```python
from build123d import *

# Parameters (mm, degrees)
F0_R         = 2.8
F1_DEPTH     = 11
F3_DEPTH     = 2
F5_DEPTH     = 0.5
F6_DEPTH     = 0.5
F7_R         = 0.8
F8_T4_DEPTH  = 7.176254213
F8_S5_R      = 2.8
F8_T6_DEPTH  = 5
F8_T10_DEPTH = 7.240123034
F8_S11_R     = 2.8
F8_T12_DEPTH = 5
F8_T16_DEPTH = 10.9265531961
F8_S17_R     = 2.8
F8_T18_DEPTH = 7
F8_T24_DEPTH = 10.862684375
F8_S25_R     = 2.8
F8_T26_DEPTH = 7
F9_R         = 0.8


# Not quite as in the source:
# - a fillet or chamfer that OpenCascade refuses, or shapes differently, is made with other operations: its cross-section is extruded or revolved along the edge and cut away or added


with BuildPart() as f1:
    # F0 (on Top) → F1 (new body)
    with BuildSketch(Plane.XY):
        Polygon((4.8497422612, -8.4), (9.6994845224, 0), (4.8497422612, 8.4), (-4.8497422612, 8.4), (-9.6994845224, 0), (-4.8497422612, -8.4), align=None)
        with Locations((-0.031784919, 0.0747148006)):
            Circle(F0_R, mode=Mode.SUBTRACT)
    extrude(amount=F1_DEPTH)

    # F2 (on Top) → F3 (cut)
    with BuildSketch(Plane.XY):
        with BuildLine():
            Line((-6, 1.1), (-6, -1.1))
            Line((-6, -1.1), (-3.585038354, -1.1))
            ThreePointArc((-3.585038354, -1.1), (-3.75, 0), (-3.585038354, 1.1))
            Line((-3.585038354, 1.1), (-6, 1.1))
        make_face()
        with BuildLine():
            ThreePointArc((-3.585038354, 1.1), (-3.75, 0), (-3.585038354, -1.1))
            Line((-3.585038354, -1.1), (3.585038354, -1.1))
            ThreePointArc((3.585038354, -1.1), (3.7085302903, -0.556150237), (3.75, 0))
            ThreePointArc((3.75, 0), (3.7085302903, 0.556150237), (3.585038354, 1.1))
            Line((3.585038354, 1.1), (-3.585038354, 1.1))
        make_face()
        with BuildLine():
            ThreePointArc((3.75, 0), (3.7085302903, -0.556150237), (3.585038354, -1.1))
            Line((3.585038354, -1.1), (6, -1.1))
            Line((6, -1.1), (6, 1.1))
            Line((6, 1.1), (3.585038354, 1.1))
            ThreePointArc((3.585038354, 1.1), (3.7085302903, 0.556150237), (3.75, 0))
        make_face()
    extrude(amount=F3_DEPTH, mode=Mode.SUBTRACT)

    # F4 (on face) → F5 (join)
    with BuildSketch(Plane(origin=(0, 0, 0), x_dir=(1, 0, 0), z_dir=(0, 0, -1))):
        with BuildLine():
            Line((2.509876966, 1.1), (3.585038354, 1.1))
            ThreePointArc((3.585038354, 1.1), (0, 3.75), (-3.585038354, 1.1))
            Line((-3.585038354, 1.1), (-2.5734468039, 1.1))
            ThreePointArc((-2.5734468039, 1.1), (-0.031784919, 2.7252851994), (2.509876966, 1.1))
        make_face()
    extrude(amount=F5_DEPTH)

    # F4 (on face) → F6 (join)
    with BuildSketch(Plane(origin=(0, 0, 0), x_dir=(1, 0, 0), z_dir=(0, 0, -1))):
        with BuildLine():
            ThreePointArc((-3.585038354, -1.1), (0, -3.75), (3.585038354, -1.1))
            Line((3.585038354, -1.1), (2.573745787, -1.1))
            ThreePointArc((2.573745787, -1.1), (-0.031784919, -2.8747148006), (-2.637315625, -1.1))
            Line((-2.637315625, -1.1), (-3.585038354, -1.1))
        make_face()
    extrude(amount=F6_DEPTH)

    # F7
    f7_edges = [f1.edges().sort_by_distance(p)[0] for p in [
        (-0.031785, 2.874715, -0.5),
        (-0.031785, -2.725285, -0.5),
    ]]
    fillet(f7_edges, radius=F7_R)

    # F8: fillet of radius 1.5 on 4 edges, made by hand


with BuildPart() as f8_tool2:
    # F8_s3 → F8_t4 (new body)
    with BuildSketch(Plane.YZ.offset(6)):
        with BuildLine():
            ThreePointArc((1.1, 0.5), (0.6606601718, 1.5606601718), (-0.4, 2))
            Line((-0.4, 2), (1.1, 2))
            Line((1.1, 2), (1.1, 0.5))
        make_face()
    extrude(amount=-F8_T4_DEPTH)

    # F8_s5 → F8_t6 (cut, symmetric)
    with BuildSketch(Plane.XY.offset(1.2)):
        with Locations((-0.031784919, 0.0747148006)):
            Circle(F8_S5_R)
    extrude(amount=F8_T6_DEPTH, both=True, mode=Mode.SUBTRACT)


with BuildPart() as f1_1:
    add(f1.part)

    # F8_t1: union F8_tool2
    add(f8_tool2.part)


with BuildPart() as f8_tool8:
    # F8_s9 → F8_t10 (new body)
    with BuildSketch(Plane.YZ.offset(-1.240123034)):
        with BuildLine():
            ThreePointArc((0.4, 2), (-0.6606601718, 1.5606601718), (-1.1, 0.5))
            Line((-1.1, 0.5), (-1.1, 2))
            Line((-1.1, 2), (0.4, 2))
        make_face()
    extrude(amount=F8_T10_DEPTH)

    # F8_s11 → F8_t12 (cut, symmetric)
    with BuildSketch(Plane.XY.offset(1.2)):
        with Locations((-0.031784919, 0.0747148006)):
            Circle(F8_S11_R)
    extrude(amount=F8_T12_DEPTH, both=True, mode=Mode.SUBTRACT)


with BuildPart() as f1_2:
    add(f1_1.part)

    # F8_t7: union F8_tool8
    add(f8_tool8.part)


with BuildPart() as f8_tool14:
    # F8_s15 → F8_t16 (new body)
    with BuildSketch(Plane.YZ.offset(-9.75)):
        with BuildLine():
            ThreePointArc((0.4, 2), (-0.6606601718, 1.5606601718), (-1.1, 0.5))
            Line((-1.1, 0.5), (-1.1, 2))
            Line((-1.1, 2), (0.4, 2))
        make_face()
    extrude(amount=F8_T16_DEPTH)

    # F8_s17 → F8_t18 (cut, symmetric)
    with BuildSketch(Plane.XY.offset(1.2)):
        with Locations((-0.031784919, 0.0747148006)):
            Circle(F8_S17_R)
    extrude(amount=F8_T18_DEPTH, both=True, mode=Mode.SUBTRACT)

    split(bisect_by=Plane(origin=(-7.2746133918, -4.2, 0), x_dir=(0, 0, 1), z_dir=(0.8660254038, 0.5, 0)), keep=Keep.TOP)

    split(bisect_by=Plane(origin=(-7.2746133918, 4.2, 0), x_dir=(0, 0, 1), z_dir=(0.8660254038, -0.5, 0)), keep=Keep.TOP)


with BuildPart() as f1_3:
    add(f1_2.part)

    # F8_t13: union F8_tool14
    add(f8_tool14.part)


with BuildPart() as f8_tool22:
    # F8_s23 → F8_t24 (new body)
    with BuildSketch(Plane.YZ.offset(1.112684375)):
        with BuildLine():
            ThreePointArc((1.1, 0.5), (0.6606601718, 1.5606601718), (-0.4, 2))
            Line((-0.4, 2), (1.1, 2))
            Line((1.1, 2), (1.1, 0.5))
        make_face()
    extrude(amount=-F8_T24_DEPTH)

    # F8_s25 → F8_t26 (cut, symmetric)
    with BuildSketch(Plane.XY.offset(1.2)):
        with Locations((-0.031784919, 0.0747148006)):
            Circle(F8_S25_R)
    extrude(amount=F8_T26_DEPTH, both=True, mode=Mode.SUBTRACT)

    split(bisect_by=Plane(origin=(-7.2746133918, -4.2, 0), x_dir=(0, 0, 1), z_dir=(0.8660254038, 0.5, 0)), keep=Keep.TOP)

    split(bisect_by=Plane(origin=(-7.2746133918, 4.2, 0), x_dir=(0, 0, 1), z_dir=(0.8660254038, -0.5, 0)), keep=Keep.TOP)


with BuildPart() as f1_4:
    add(f1_3.part)

    # F8_t21: union F8_tool22
    add(f8_tool22.part)

    # F9
    f9_edges = [f1_4.edges().sort_by_distance(p)[0] for p in [
        (0, -8.4, 11),
        (7.274613, -4.2, 11),
        (7.274613, 4.2, 11),
        (0, 8.4, 11),
        (-7.274613, 4.2, 11),
        (-7.274613, -4.2, 11),
    ]]
    fillet(f9_edges, radius=F9_R)


solid = f1_4.part
```
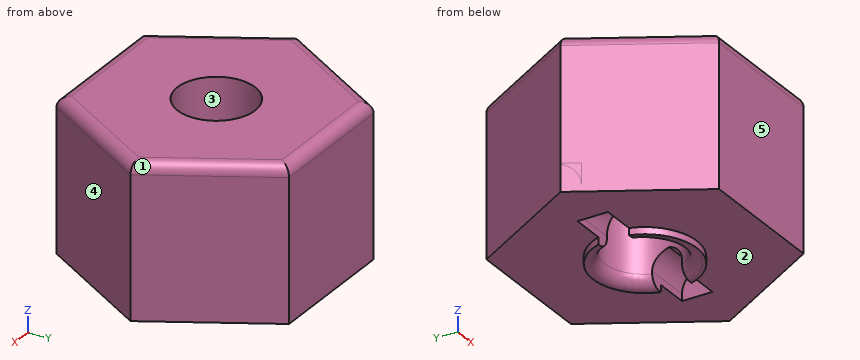
Could you check a few things on this model? Use its own coordinates, in mm. Face numbers are marked on the shaded views. A direction names the side the tool comes from. Round coordinates to 2 decimals unless told otherwise and drop trailing zeros. Loops run counter-clockwise (first coordinate to the right, second up) from the corner with the lowest first, then second, coordinate; pieces in that order, holes last. Notation, with made-up numbers: (-22, 54) -> (-8, 54) arc R15 cw to (-8, 65) -> close; hole circle Ø6 at (64.5, -25). An arc over 180 degrees is marked (long way). One line per question, with ' | ' between items.
(1) Thinking about a two-plate mould opening in X: for the marked faces 3, 4 and 5, which applies, released by +X, released by -X, zero draft, split by the parting line, or undercut?
Model answer:
face 3: undercut | face 4: released by +X | face 5: zero draft
(2) If we section it at B-B on z = 1.25: List the corners of the cut face in (x, y) for me, and give its area (3 significant figures).
Model answer:
outline: (-9.7, 0) -> (-4.85, -8.4) -> (4.85, -8.4) -> (9.7, 0) -> (4.85, 8.4) -> (-4.85, 8.4) -> close; hole (-6, -0.9) -> (-2.66, -0.9) arc R2.8 ccw to (2.59, -0.9) -> (6, -0.9) -> (6, 0.9) -> (2.64, 0.9) arc R2.8 ccw to (-2.71, 0.9) -> (-6, 0.9) -> close | area: 208 mm^2
(3) For pin 1 Ø5 at (y, z) = (1, 3.5) entering from +X; pin 2 Ø1 at (y, z) = (2, 1.5) entering from +X; pin 3 Ø1 at (y, z) = (-1, 1) entering from +X, each with a flat end and sliding along its axis, tell me the tip position at first contact or that it passes through.
Model answer:
pin 1: stops at x = 9.7 | pin 2: stops at x = 8.83 | pin 3: stops at x = 9.41
(4) If I drill on probe 1 along Z at (x, y) = (6.25, 4); probe 2 along X at (y, z) = (-1.75, 5.25); probe 3 along Y at (x, z) = (0.75, 7.75), over which ranges is the centre line in solid material (lowest first)?
Model answer:
probe 1: z = 0 to 11 | probe 2: x = -8.69 to -2.16, 2.09 to 8.69 | probe 3: y = -8.4 to -2.61, 2.76 to 8.4
(5) For the marked faces 1 and 2, which set-ups out of +Z, -Z, +X, -X, +Y, -Y let a thin tool reach every point of the face, with its end or its side?
Model answer:
face 1: +Z, +X, +Y | face 2: -Z
(6) If we section it at A-A on z = 8: List the corners of the cut face in (x, y) for me, and give its area (3 significant figures).
Model answer:
outline: (-9.7, 0) -> (-4.85, -8.4) -> (4.85, -8.4) -> (9.7, 0) -> (4.85, 8.4) -> (-4.85, 8.4) -> close; hole circle Ø5.6 at (-0.03, 0.07) | area: 220 mm^2
